Autodesk Inventor part; units mm, degrees
ref_plane "YZ Plane" through (0, 0, 0) normal (1, 0, 0) x (0, 1, 0)
ref_plane "XZ Plane" through (0, 0, 0) normal (0, 1, 0) x (-1, 0, 0)
ref_plane "XY Plane" through (0, 0, 0) normal (0, 0, 1) x (1, 0, 0)
sketch "Sketch1" plane through (0, 0, 0) normal (1, 0, 0) x (0, 1, 0)
  circle A0 centre (0, 0) radius 12.5
  line L0 (0, 0) -> (0, -55) construction
  circle A1 centre (0, -55) radius 12.5
  line L1 (0, -55) -> (35.3553, -90.3553) construction
  circle A2 centre (35.3553, -90.3553) radius 10
  line L2 (10.9114, -6.0985) -> (10.9114, -48.9015)
  line L3 (-9.0886, -8.5818) -> (-9.0886, -46.4182)
  line L4 (40.0876, -81.5459) -> (12.4612, -54.0158)
  line L5 (0.7049, -67.4801) -> (25.5516, -92.3268)
  dimension "d0" = 25
  dimension "d1" = 55
  dimension "d2" = 25
  dimension "d3" = 50
  dimension "d4" = 20
  dimension "d5" = 20
  dimension "d7" = 45
  dimension "d8" = 0.1
extrude "Extrusion1" add sketch "Sketch1" along normal mid plane 8
sketch "Sketch2" plane through (4, 0, 0) normal (1, 0, 0) x (0, 0, -1)
  circle A0 centre (0, 0) radius 12.5
  line L0 (0, 0) -> (55, 0) construction
  circle A1 centre (55, 0) radius 12.5
  line L1 (55, 0) -> (90.3553, 35.3553)
  circle A2 centre (90.3553, 35.3553) radius 10
  dimension "d11" = 25
  dimension "d12" = 55
  dimension "d13" = 25
  dimension "d14" = 50
  dimension "d15" = 45
  dimension "d16" = 20
extrude "Extrusion2" add sketch "Sketch2" along normal blind 2
sketch "Sketch3" plane through (-4, 0, 0) normal (-1, 0, 0) x (0, 0, 1)
  line L0 (0, 0) -> (-55, 0) construction
  line L1 (-55, 0) -> (-90.3553, 35.3553) construction
  circle A0 centre (-90.3553, 35.3553) radius 10
  circle A1 centre (-55, 0) radius 12.5
  circle A2 centre (0, 0) radius 12.5
  dimension "d19" = 55
  dimension "d20" = 50
  dimension "d21" = 45
  dimension "d22" = 20
  dimension "d23" = 25
  dimension "d24" = 25
extrude "Extrusion3" add sketch "Sketch3" along normal blind 2
sketch "Sketch4" plane through (6, 0, 0) normal (1, 0, 0) x (0, 0, -1)
  circle A0 centre (0, 0) radius 6
  line L0 (0, 0) -> (55, 0) construction
  line L1 (55, 0) -> (90.3553, 35.3553) construction
  line L2 (49, -6) -> (61, -6)
  line L3 (61, -6) -> (61, 6)
  line L4 (61, 6) -> (49, 6)
  line L5 (49, 6) -> (49, -6)
  line L6 (49, -6) -> (61, 6) construction
  line L7 (61, -6) -> (49, 6) construction
  circle A1 centre (90.3553, 35.3553) radius 5
  dimension "d27" = 12
  dimension "d28" = 55
  dimension "d29" = 50
  dimension "d30" = 45
  dimension "d31" = 12
  dimension "d32" = 12
  dimension "d33" = 10
extrude "Extrusion4" cut sketch "Sketch4" against normal through all
Model file for the job. Use its own axes, mm. A direction names the side the tool comes from. Give positions to 0.01 mm unless a question says otherwise; leave off trailing zeros. Write each loop counter-clockwise with the first axis right and the second up, starting at its lowest first coordinate (ties: lowest second). Pieces come first, ordered by that corner, then holes. Notation, with made-up numbers: (-4.5, -20) -> (19.5, -20) arc R24 ccw to (19.5, -9) -> close; hole circle Ø6 at (29, 45). An arc over 180 degrees is marked (long way). Use CSV: the item, a comma, the result in double quotes. Start each with the question number.
1) Cut at C-C on z = -2. List the corners of the cut face in (x, y).
2) Cut at D-D on z = -34. List the corners of the cut face in (x, y), plus the area to 3 significant figures.
3) Two-plate mould, pull along Z, no slides. Class faces 4 (the cylindrical face through (-0.084, 40.915, -98.667)), 5 (the cylindrical face through (0.084, 33.44, -94.974)), 6 (the flat face through (0, -9.089, -27)), 7 (the flat face through (-4, 19, -73)): released by +Z, released by -Z, zero draft, split by the parting line, or undercut.
4) Pin check, flat tips, straight feed: P1, Ø6.5, axis at x = 0, z = -32, coming from the +Y side; P2, Ø3, axis at x = 0, z = -67.5, coming from the +Y side; P3, Ø19, axis at y = 28, z = -64.5, coming from the -X side. Stop position of each tip, or through.
5) Drill centre lines: L1, parallel to Z at x = 4.25, y = -3; L2, parallel to Z at x = 2.5, y = 1; L3, parallel to Z at x = -5.25, y = 7. Where is each one in solid material? Low to high.
6) Cut at A-A on z = -56. List the corners of the cut face in (x, y).
7) Cut at B-B on x = 0.5. List the corners of the cut face in (y, z).
8) Tool access for faces 1 (the flat face through (0, 6, -55)), 2 (the flat face through (4, 19, -73)), 3 (the cylindrical face through (-1.417, -5.523, -66.214)): list every direction of +Z, -Z, +X, -X, +Y, -Y with a clear straight run to the whole face (end or side of a thin tool).
Final values:
1,outline,"(-6, -12.34) -> (6, -12.34) -> (6, -5.66) -> (-6, -5.66) -> close; (-6, 5.66) -> (6, 5.66) -> (6, 12.34) -> (-6, 12.34) -> close"
2,outline,"(-4, -9.09) -> (4, -9.09) -> (4, 10.91) -> (-4, 10.91) -> close"
2,area,"160 mm2"
3,face 4,"split by the parting line"
3,face 5,"undercut"
3,face 6,"undercut"
3,face 7,"zero draft"
4,P1,"stops at y = 10.91"
4,P2,"stops at y = 27.5"
4,P3,"stops at x = -4"
5,L1,"z = -67.13 to -61, -49 to -42.87, -12.13 to -5.2, 5.2 to 12.13"
5,L2,"z = -67.78 to -61, -49 to -5.92, 5.92 to 12.46"
5,L3,"z = -65.36 to -44.64, -10.36 to 10.36"
6,outline,"(-6, -12.46) -> (6, -12.46) -> (6, -6) -> (-6, -6) -> close; (-6, 6) -> (6, 6) -> (6, 12.46) -> (4, 12.46) -> (4, 14.45) -> (-4, 14.45) -> (-4, 12.46) -> (-6, 12.46) -> close"
7,outline,"(-9.09, -46.42) arc R12.5 ccw to (0.7, -67.48) -> (25.55, -92.33) arc R10 ccw (long way) to (40.09, -81.55) -> (12.46, -54.02) arc R12.5 ccw to (10.91, -48.9) -> (10.91, -6.1) arc R12.5 ccw (long way) to (-9.09, -8.58) -> close; hole (-6, -61) -> (6, -61) -> (6, -49) -> (-6, -49) -> close; hole circle Ø12 at (0, 0); hole circle Ø10 at (35.36, -90.36)"
8,face 1,"+X, -X"
8,face 2,"+X"
8,face 3,"none"
